Read the model definition and answer for the solid it produces. Units are mm, in the model's axes. Face numbers are marked on the shaded views. A direction names the side the tool comes from. Give positions to 0.01 mm unless a question says otherwise; leave off trailing zeros. Write each loop counter-clockwise with the first axis right and the second up, starting at its lowest first coordinate (ties: lowest second). Pieces come first, ordered by that corner, then holes. Notation, with made-up numbers: M 34,86 L 69,86 A34 ccw 69,125 Z; hole C -3,-12.5 d11. An arc over 180 degrees is marked long. Use a Markdown table: item, result. Add a question column.
Item 1: A cutting plane is placed at B-B on z = 7. Determine the outline of the cut face in (x, y), then the cut area to 3 significant figures.
Item 2: Consider probe 1 along Y at (x, z) = (9.5, 11); probe 2 along Y at (x, z) = (-7.5, 18.25) (3 decimals); probe 3 along X at (y, z) = (-1.75, 1.75). Determine where each line is inside the solid, lowest interval first. Write a range as [from, to].
Item 3: A cutting plane is placed at C-C on x = 9.5. Determine the outline of the cut face in (y, z), then the cut area to 3 significant figures.
Item 4: A cutting plane is placed at D-D on y = 0. Determine the outline of the cut face in (x, z).
Item 5: A cutting plane is placed at A-A on x = -2.75. Determine the outline of the cut face in (y, z), then the cut area to 3 significant figures.
Item 6: The mould has two halves that part along Y. Classify the marked faces 1, 2 and 3: pulls with the +Y half, pulls with the -Y half, needs draft (parallel to the pull), parting line crosses it, or undercut.
Item 7: For the marked faces 4 and 5, determine the directions among +Z, -Z, +X, -X, +Y, -Y from which every point of the face is accessible in a straight line to the end or side of a thin tool.
Item 8: Given P1, Ø2, axis at y = -1, z = 16.5, coming from the +X side, flat-ended and moving along its own axis, determine where the tip first touches the part or whether it passes through.
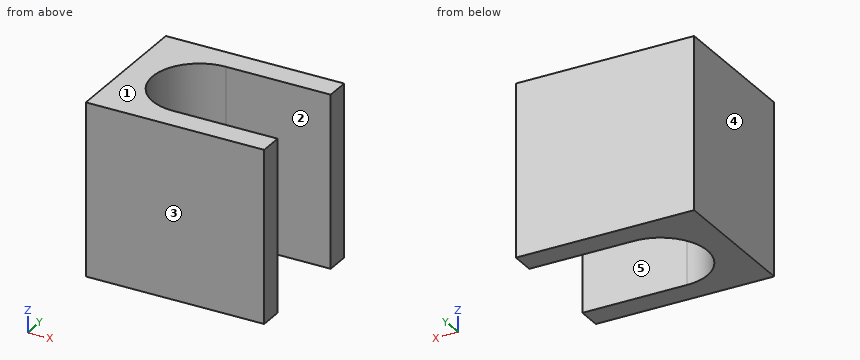
from build123d import *

# Parameters (mm, degrees)
SKETCH_1_24X19_W         = 19
SKETCH_1_24X19_H         = 24
EXTRUDE_1_33_DEPTH       = 33
CUT_EXTRUDE_2_REACH      = 38.377
CUT_EXTRUDE_4_2_DEPTH    = 1.9
CUT_EXTRUDE_6_3_REACH    = 29.71
SKETCH_7_5_W             = 24
SKETCH_7_5_H             = 19
EXTRUDE_7_DEPTH          = 5
CUT_EXTRUDE_10_4_REACH   = 41.925
SKETCH_11_W              = 8.5
SKETCH_11_H              = 3.1
CUT_EXTRUDE_11_5_DEPTH   = 4.9
SKETCH_11D1_W            = 6
SKETCH_11D1_H            = 3.1
CUT_EXTRUDE_11D1_6_DEPTH = 10
CUT_EXTRUDE_12_9_REACH   = 31.655
CUT_EXTRUDE_11_DEPTH     = 3.5
SKETCH_5903_W            = 53.98
SKETCH_5903_H            = 19
CUT_EXTRUDE_12_DEPTH     = 1
CUT_EXTRUDE_13_DEPTH     = 40.102429623
CUT_EXTRUDE_15_REACH     = 33.036
SKETCH_5021_R            = 3.5
EXTRUDE_2_DEPTH          = 0.4
SKETCH_7445_W            = 0.8
SKETCH_7445_H            = 3.1
EXTRUDE_3_DEPTH          = 19
CUT_EXTRUDE_16_DEPTH     = 32.036269144
SKETCH_14_W              = 24
SKETCH_14_H              = 19
CUT_EXTRUDE_19_DEPTH     = 28.710286942


with BuildPart() as part:
    # 1底部方形_24x19 → 1凸台-拉伸_高33 (new body)
    with BuildSketch(Plane(origin=(0, 0, 0), x_dir=(0, 1, 0), z_dir=(0, 0, 1))):
        Rectangle(SKETCH_1_24X19_W, SKETCH_1_24X19_H)
    extrude(amount=EXTRUDE_1_33_DEPTH)

    # 2吸嘴停靠渐变槽 → 2切除-拉伸 (cut, up to next)
    with BuildSketch(Plane.XY.offset(33), mode=Mode.PRIVATE) as cut_extrude_2_sk1:
        with BuildLine():
            Line((12, -5.1), (12, 5.1))
            Line((12, 5.1), (-1.9, 5.1))
            add(Edge.make_bspline(
                [(-5.213938048, 3.830222216), (-3.829124073, 5.093205317), (-1.9, 5.1)],
                knots=[0, 0, 0, 1, 1, 1], degree=2))
            ThreePointArc((-5.213938048, 3.830222216), (-7, 0), (-5.213938048, -3.830222216))
            add(Edge.make_bspline(
                [(-5.213938048, -3.830222216), (-3.829124073, -5.093205317), (-1.9, -5.1)],
                knots=[0, 0, 0, 1, 1, 1], degree=2))
            Line((-1.9, -5.1), (12, -5.1))
        make_face()
    cut_extrude_2_tool1 = extrude(cut_extrude_2_sk1.sketch, amount=-CUT_EXTRUDE_2_REACH, mode=Mode.PRIVATE) & part.part
    add(cut_extrude_2_tool1.solids().sort_by_distance((3.017719, 0, 33))[0], mode=Mode.SUBTRACT)

    # 4反光板停靠槽 → 4切除-拉伸2 (cut)
    with BuildSketch(Plane.XY.offset(25)):
        with BuildLine():
            Line((-0.7, 8.4), (12, 8.4))
            Line((12, 8.4), (12, -8.4))
            Line((12, -8.4), (-0.7, -8.4))
            ThreePointArc((-0.7, -8.4), (-10.5, 0), (-0.7, 8.4))
        make_face()
    extrude(amount=-CUT_EXTRUDE_4_2_DEPTH, mode=Mode.SUBTRACT)

    # 6反光板小圆柱 → 6切除-拉伸3 (cut, up to next)
    with BuildSketch(Plane.XY.offset(23.1), mode=Mode.PRIVATE) as cut_extrude_6_3_sk1:
        with BuildLine():
            Line((-2.1, -6.3), (12, -6.3))
            Line((12, -6.3), (12, 6.3))
            Line((12, 6.3), (-2.1, 6.3))
            ThreePointArc((-2.1, 6.3), (-8.4, 0), (-2.1, -6.3))
        make_face()
    cut_extrude_6_3_tool1 = extrude(cut_extrude_6_3_sk1.sketch, amount=-CUT_EXTRUDE_6_3_REACH, mode=Mode.PRIVATE) & part.part
    add(cut_extrude_6_3_tool1.solids().sort_by_distance((2.424095, 0, 23.1))[0], mode=Mode.SUBTRACT)

    # 7草图5 → 7凸台-拉伸_底板厚度 (add)
    with BuildSketch(Plane(origin=(0, 0, 0), x_dir=(1, 0, 0), z_dir=(0, 0, -1))):
        Rectangle(SKETCH_7_5_W, SKETCH_7_5_H)
    extrude(amount=-EXTRUDE_7_DEPTH)

    # 10切除-拉伸4: up to this face of the body (flat: up to its plane)
    cut_extrude_10_4_end = Plane(part.part.faces().sort_by_distance((0, -9.5, 16.5))[0])
    # Sketch 10 → 10切除-拉伸4 (cut, up to the picked face)
    with BuildSketch(Plane(origin=(0, 9.5, 0), x_dir=(-1, 0, 0), z_dir=(0, 1, 0)), mode=Mode.PRIVATE) as cut_extrude_10_4_sk1:
        Polygon((-12, 31.162738066), (-12, 33), (9, 33), align=None)
    cut_extrude_10_4_tool1 = split(extrude(cut_extrude_10_4_sk1.sketch, amount=-CUT_EXTRUDE_10_4_REACH, mode=Mode.PRIVATE), bisect_by=cut_extrude_10_4_end, keep=Keep.BOTH, mode=Mode.PRIVATE)
    add(cut_extrude_10_4_tool1.solids().sort_by(Axis((5, 9.5, 32.387579), (0, -1, 0)))[0], mode=Mode.SUBTRACT)

    # Sketch 11 → 11切除-拉伸5 (cut)
    with BuildSketch(Plane(origin=(-12, 0, 0), x_dir=(0, -1, 0), z_dir=(-1, 0, 0))):
        with Locations((-5.25, 26.95)):
            Rectangle(SKETCH_11_W, SKETCH_11_H)
        with Locations((5.25, 26.95)):
            Rectangle(SKETCH_11_W, SKETCH_11_H)
    extrude(amount=-CUT_EXTRUDE_11_5_DEPTH, mode=Mode.SUBTRACT)

    # 11d1_磁铁开窗 → 11d1切除-拉伸6 (cut)
    with BuildSketch(Plane(origin=(-12, 0, 0), x_dir=(0, -1, 0), z_dir=(-1, 0, 0))):
        with Locations((0, 26.95)):
            Rectangle(SKETCH_11D1_W, SKETCH_11D1_H)
    extrude(amount=-CUT_EXTRUDE_11D1_6_DEPTH, mode=Mode.SUBTRACT)

    # 12切除薄壁 → 12切除-拉伸9 (cut, up to next)
    with BuildSketch(Plane.XY.offset(25.4), mode=Mode.PRIVATE) as cut_extrude_12_9_sk1:
        with BuildLine():
            Line((-0.7, 8.4), (-0.7, -8.4))
            ThreePointArc((-0.7, -8.4), (-10.5, 0), (-0.7, 8.4))
        make_face()
    cut_extrude_12_9_tool1 = extrude(cut_extrude_12_9_sk1.sketch, amount=-CUT_EXTRUDE_12_9_REACH, mode=Mode.PRIVATE) & part.part
    add(cut_extrude_12_9_tool1.solids().sort_by_distance((-4.916056, 0, 25.4))[0], mode=Mode.SUBTRACT)

    # Sketch 5393 → 切除-拉伸11 (cut)
    with BuildSketch(Plane.XY.offset(33)):
        with BuildLine():
            Line((-2.099999748, 6.5), (12, 6.5))
            Line((12, 6.5), (12, -6.5))
            Line((12, -6.5), (-2.099999748, -6.5))
            ThreePointArc((-2.099999748, -6.5), (-8.6, 0), (-2.099999748, 6.5))
        make_face()
    extrude(amount=-CUT_EXTRUDE_11_DEPTH, mode=Mode.SUBTRACT)

    # Sketch 5903 → 切除-拉伸12 (cut)
    with BuildSketch(Plane.XY.offset(33)):
        with Locations((14.99, 0)):
            Rectangle(SKETCH_5903_W, SKETCH_5903_H)
    extrude(amount=-CUT_EXTRUDE_12_DEPTH, mode=Mode.SUBTRACT)

    # Sketch 6208 → 切除-拉伸13 (cut, through all)
    with BuildSketch(Plane.XZ.offset(9.5)):
        Polygon((2.430052303, 32), (12, 31.162738066), (12, 28.826114347), (-6, 32), align=None)
    extrude(amount=-CUT_EXTRUDE_13_DEPTH, mode=Mode.SUBTRACT)

    # Sketch 5021 → 切除-拉伸15 (cut, up to next)
    with BuildSketch(Plane.XY.offset(5), mode=Mode.PRIVATE) as cut_extrude_15_sk1:
        with Locations((2, 0)):
            Circle(SKETCH_5021_R)
    cut_extrude_15_tool1 = extrude(cut_extrude_15_sk1.sketch, amount=-CUT_EXTRUDE_15_REACH, mode=Mode.PRIVATE) & part.part
    add(cut_extrude_15_tool1.solids().sort_by_distance((2, 0, 5))[0], mode=Mode.SUBTRACT)

    # Sketch 6983 → 凸台-拉伸2 (add)
    with BuildSketch(Plane(origin=(0, 0, 25.4), x_dir=(1, 0, 0), z_dir=(0, 0, -1))):
        with BuildLine():
            Line((-7.1, -3), (-7.1, -6.8))
            ThreePointArc((-7.1, -6.8), (-4.061552813, -8.246211251), (-0.7, -8.4))
            Line((-0.7, -8.4), (-0.7, -5.1))
            Line((-0.7, -5.1), (-1.9, -5.1))
            add(Edge.make_bspline(
                [(-1.9, -5.1), (-3.829124073, -5.093205317), (-5.213938048, -3.830222216)],
                knots=[0, 0, 0, 1, 1, 1], degree=2))
            ThreePointArc((-5.213938048, -3.830222216), (-5.630777158, -3.437652866), (-6, -3))
            Line((-6, -3), (-7.1, -3))
        make_face()
        with BuildLine():
            Line((-7.1, 3), (-6, 3))
            ThreePointArc((-6, 3), (-5.630777158, 3.437652866), (-5.213938048, 3.830222216))
            add(Edge.make_bspline(
                [(-5.213938048, 3.830222216), (-3.829124073, 5.093205317), (-1.9, 5.1)],
                knots=[0, 0, 0, 1, 1, 1], degree=2))
            Line((-1.9, 5.1), (-0.7, 5.1))
            Line((-0.7, 5.1), (-0.7, 8.4))
            ThreePointArc((-0.7, 8.4), (-4.061552813, 8.246211251), (-7.1, 6.8))
            Line((-7.1, 6.8), (-7.1, 3))
        make_face()
    extrude(amount=EXTRUDE_2_DEPTH)

    # Sketch 7445 → 凸台-拉伸3 (add)
    with BuildSketch(Plane.XZ.offset(9.5)):
        with Locations((-11.6, 26.95)):
            Rectangle(SKETCH_7445_W, SKETCH_7445_H)
    extrude(amount=-EXTRUDE_3_DEPTH)

    # 草图13 → 切除-拉伸16 (cut, through all)
    with BuildSketch(Plane.XY.offset(5)):
        with BuildLine():
            Line((-2.1, -6.3), (12, -6.3))
            Line((12, -6.3), (12, 6.3))
            Line((12, 6.3), (-2.1, 6.3))
            ThreePointArc((-2.1, 6.3), (-8.4, 0), (-2.1, -6.3))
        make_face()
    extrude(amount=-CUT_EXTRUDE_16_DEPTH, mode=Mode.SUBTRACT)

    # 草图14 → 切除-拉伸19 (cut, through all)
    with BuildSketch(Plane.XY.offset(23.1)):
        Rectangle(SKETCH_14_W, SKETCH_14_H)
    extrude(amount=CUT_EXTRUDE_19_DEPTH, mode=Mode.SUBTRACT)


solid = part.part
Filled in:
| question | item | result |
|---|---|---|
| 1 | outline | M -12,-9.5 L 12,-9.5 L 12,-6.3 L -2.1,-6.3 A6.3 cw -2.1,6.3 L 12,6.3 L 12,9.5 L -12,9.5 Z |
| 1 | area | 216 mm² |
| 2 | probe 1 | [-9.5, -6.3], [6.3, 9.5] |
| 2 | probe 2 | [-9.5, -3.245], [3.245, 9.5] |
| 2 | probe 3 | [-12, -8.15] |
| 3 | outline | M -9.5,0 L -6.3,0 L -6.3,23.1 L -9.5,23.1 Z; M 6.3,0 L 9.5,0 L 9.5,23.1 L 6.3,23.1 Z |
| 3 | area | 148 mm² |
| 4 | outline | M -12,0 L -8.4,0 L -8.4,23.1 L -12,23.1 Z |
| 5 | outline | M -9.5,0 L -6.27,0 L -6.27,23.1 L -9.5,23.1 Z; M 6.27,0 L 9.5,0 L 9.5,23.1 L 6.27,23.1 Z |
| 5 | area | 149 mm² |
| 6 | face 1 | needs draft |
| 6 | face 2 | undercut |
| 6 | face 3 | pulls with the -Y half |
| 7 | face 4 | +Z, -Z, -X, +Y, -Y |
| 7 | face 5 | +Z, -Z, +X |
| 8 | P1 | x = -8.07 |
